Input: part model. Units: mm. Frame: model coordinates. A direction names the side the tool comes from. Round coordinates to 2 decimals unless told otherwise and drop trailing zeros. Write each loop counter-clockwise with the first axis right and the second up, starting at its lowest first coordinate (ties: lowest second). Pieces come first, ordered by that corner, then holes. Notation, with made-up numbers: (54, -1.75) - (100, -1.75) arc R25 ccw to (100, 13.25) - close; hole circle Ø1 at (44.25, 62.25). An arc over 180 degrees is marked (long way). Use one line per item in the form item = value.
```python
from build123d import *

# Parameters (mm, degrees)
SKETCH2_R           = 12.065
BOSS_EXTRUDE1_DEPTH = 2.54
BOSS_EXTRUDE2_DEPTH = 7.62
CIRPATTERN1_COUNT   = 4
SKETCH4_R           = 1.778
CUT_EXTRUDE1_DEPTH  = 7.62
CIRPATTERN2_COUNT   = 4
FILLET1_R           = 1.27


with BuildPart() as part:
    # Sketch2 → Boss-Extrude1 (new body)
    with BuildSketch(Plane(origin=(0, 0, 0), x_dir=(1, 0, 0), z_dir=(0, 1, 0))):
        with Locations(Location((0, 0, 0), (0, 0, 270))):
            Circle(SKETCH2_R)
    extrude(amount=BOSS_EXTRUDE1_DEPTH)

    # Sketch3 → Boss-Extrude2 (add)
    with BuildSketch(Plane(origin=(0, 0, 0), x_dir=(1, 0, 0), z_dir=(0, 1, 0))):
        with BuildLine():
            Line((-11.4476253, 3.81), (-19.0676253, 3.81))
            Line((-19.0676253, 3.81), (-19.0676253, -3.81))
            Line((-19.0676253, -3.81), (-11.4476253, -3.81))
            ThreePointArc((-11.4476253, -3.81), (-12.065, 0), (-11.4476253, 3.81))
        make_face()
    boss_extrude2 = extrude(amount=BOSS_EXTRUDE2_DEPTH)

    # CirPattern1: Boss-Extrude2 ×4 about axis
    cirpattern1_axis = Axis((0, 0, 0), (0, 1, 0))
    for i in range(1, CIRPATTERN1_COUNT):
        add(boss_extrude2.rotate(cirpattern1_axis, i * 360 / CIRPATTERN1_COUNT))

    # Sketch4 → Cut-Extrude1 (cut)
    with BuildSketch(Plane.XY.offset(3.81)):
        with Locations((-15.2576253, 3.81)):
            Circle(SKETCH4_R)
    cut_extrude1 = extrude(amount=-CUT_EXTRUDE1_DEPTH, mode=Mode.SUBTRACT)

    # CirPattern2: Cut-Extrude1 ×4 about axis
    cirpattern2_axis = Axis((0, 2.54, 0), (0, -1, 0))
    for i in range(1, CIRPATTERN2_COUNT):
        add(cut_extrude1.rotate(cirpattern2_axis, i * 360 / CIRPATTERN2_COUNT), mode=Mode.SUBTRACT)

    # Fillet1
    fillet1_edges = [part.edges().sort_by_distance(p)[0] for p in [
        (8.531243315, 0, 8.531243315),
        (8.531243315, 0, -8.531243315),
        (-8.531243315, 0, -8.531243315),
        (-8.531243315, 0, 8.531243315),
    ]]
    fillet(fillet1_edges, radius=FILLET1_R)


solid = part.part
```
(1) Material intervals for L1, parallel to X at y = 5.25, z = -1; L2, parallel to Z at x = -3, y = 5; L3, parallel to Y at x = -1.5, z = -7, sorted ascending.
Derived:
L1 = -19.07 to -16.3, -14.21 to -12.02, 12.02 to 14.21, 16.3 to 19.07
L2 = -19.07 to -16.58, -13.94 to -11.69, 11.69 to 13.94, 16.58 to 19.07
L3 = 0 to 2.54
(2) Cut plane A-A on y = 3.81. Count the separate pieces of the cut face and the enclosed holes in it, then the cut area to 3 significant figures.
Derived:
separate_pieces = 8
enclosed_holes = 0
area = 111 mm^2
(3) Draft query along X for faces 3 (the face through (0, 7.62, 15)), 4 (the face through (-3.81, 2, -16)), 5 (the face through (0, 2.54, 0)). Return one class per face: released by +X, released by -X, zero draft, split by the parting line, or undercut.
Derived:
face_3 = zero draft
face_4 = released by -X
face_5 = undercut
(4) Access query for faces 1 (the face through (-15, 7.62, 0)), 2 (the face through (-0.054, 5.044, -12.065)). Directions: +Z, -Z, +X, -X, +Y, -Y. A direction counts if a zero-diameter tool reaches every point of the face in a straight line with its end or side. Return the directions, or none.
Derived:
face_1 = +Z, -Z, +X, -X, +Y
face_2 = +Y
(5) Cut plane B-B on y = 6.75. Output: boundary loops of the cut face in (x, z) (3 decimals).
Derived:
outline = (-19.068, -3.81) - (-11.448, -3.81) arc R12.065 cw to (-11.448, 3.81) - (-19.068, 3.81) - close; (-3.81, -19.068) - (3.81, -19.068) - (3.81, -11.448) arc R12.065 cw to (-3.81, -11.448) - close; (-3.81, 11.448) arc R12.065 cw to (3.81, 11.448) - (3.81, 19.068) - (-3.81, 19.068) - close; (11.448, -3.81) - (19.068, -3.81) - (19.068, 3.81) - (11.448, 3.81) arc R12.065 cw to start
(6) First-contact query: pin 1 Ø4.5 at (x, y) = (15.26, 3.81) entering from -Z; pin 2 Ø4 at (y, z) = (3, -13.5) entering from -X; pin 3 Ø4 at (x, z) = (-3.5, 1.5) entering from +Y. Flat tips, straight axial feed; report the tip coordinate or a pass-through.
Derived:
pin_1 = -3.81
pin_2 = -3.81
pin_3 = 2.54
(7) Cut plane C-C on z = 0.5. Output: boundary loops of the cut face in (x, y), then the cut area to 3 significant figures.
Derived:
outline = (-19.07, 0) - (19.07, 0) - (19.07, 7.62) - (12.05, 7.62) - (12.05, 2.54) - (-12.05, 2.54) - (-12.05, 7.62) - (-19.07, 7.62) - close; hole circle Ø3.56 at (-15.26, 3.81); hole circle Ø3.56 at (15.26, 3.81)
area = 148 mm^2
